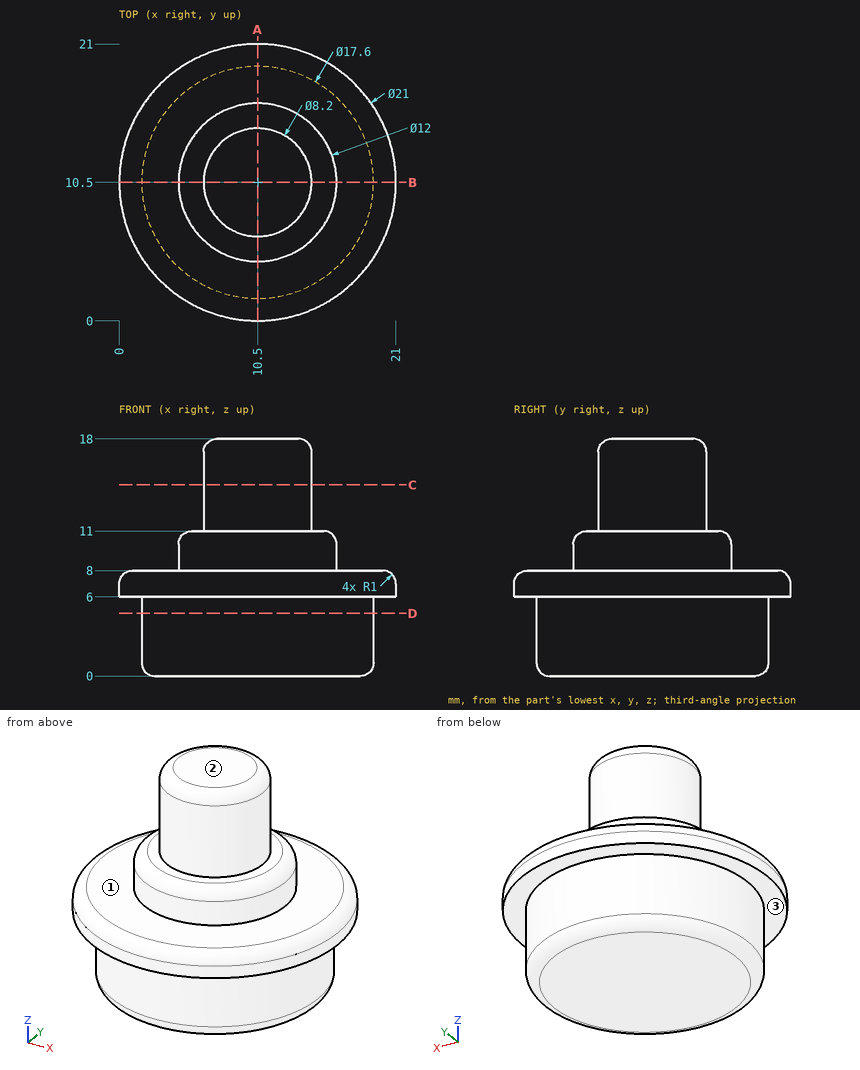
Answer from the drawing. Dimensions are ordinates in mm from the lowest x, y and z of the part. A direction names the side the tool comes from. Coordinates: 2 decimals unless noted, no trailing zeros. Loops run counter-clockwise (first coordinate to the right, second up) from the corner with the lowest first, then second, coordinate; pieces in that order, holes last. Notation, with made-up numbers: (72, 77.5) - (79, 77.5) arc R19 ccw to (79, 95.5) - close; hole circle Ø9 at (-3.75, -19.5). An arc over 180 degrees is marked (long way). Answer in a Markdown table with one row per item.
1. Which of the six approach directions +Z, -Z, +X, -X, +Y, -Y give full straight-line access (tool end or side, diameter ignored) to the marked faces 1, 2 and 3?
Conclusion:
| item | result |
|---|---|
| face 1 | +Z |
| face 2 | +Z, +X, -X, +Y, -Y |
| face 3 | -Z |
2. Given pin 1 (4 mm diameter, centred on x = 13.5, z = 12, fed in from +Y); pin 2 (2 mm diameter, centred on y = 14, z = 3.5, fed in from -X); pin 3 (5 mm diameter, centred on y = 18.5, z = 8.5, fed in from -X), each flat-ended and moving along its own axis, determine where each tip first touches the part or whether it passes through.
Conclusion:
| item | result |
|---|---|
| pin 1 | stops at y = 16.14 |
| pin 2 | stops at x = 2.06 |
| pin 3 | stops at x = 1.81 |
3. Find section C-C, the plane z = 14.5. Write down the section's boundary in (x, y), then the cut area to 3 significant figures.
Conclusion:
| item | result |
|---|---|
| outline | circle Ø8.2 at (10.5, 10.5) |
| area | 52.8 mm² |
4. Find section D-D, the plane z = 4.75. Write down the section's boundary in (x, y).
Conclusion:
| item | result |
|---|---|
| outline | circle Ø17.6 at (10.5, 10.5) |
5. Find section A-A, the plane x = 10.5. Write down the section's boundary in (y, z).
Conclusion:
| item | result |
|---|---|
| outline | (0, 6) - (1.7, 6) - (1.7, 1) arc R1 ccw to (2.7, 0) - (18.3, 0) arc R1 ccw to (19.3, 1) - (19.3, 6) - (21, 6) - (21, 7) arc R1 ccw to (20, 8) - (16.5, 8) - (16.5, 10) arc R1 ccw to (15.5, 11) - (14.6, 11) - (14.6, 17) arc R1 ccw to (13.6, 18) - (7.4, 18) arc R1 ccw to (6.4, 17) - (6.4, 11) - (5.5, 11) arc R1 ccw to (4.5, 10) - (4.5, 8) - (1, 8) arc R1 ccw to (0, 7) - close |
6. Straight lines are drawn through the part: line 1 (Z direction, x = 7.75, y = 1.5); line 2 (Z direction, x = 3.25, y = 8.5); line 3 (Y direction, x = 7.75, z = 14.5). For each, find the intervals that lie inside material, in ascending order.
Conclusion:
| item | result |
|---|---|
| line 1 | z = 6 to 8 |
| line 2 | z = 0 to 8 |
| line 3 | y = 7.46 to 13.54 |
